Read the model definition and answer for the solid it produces. Units are mm, in the model's axes. A direction names the side the tool comes from. Coordinates: 2 decimals unless noted, no trailing zeros. Write each loop counter-clockwise with the first axis right and the second up, starting at its lowest first coordinate (ties: lowest second). Pieces come first, ordered by that corner, then holes.
(1) Section A-A on y = 2 is taken. Write down the section's boundary in (x, z), then the cut area to 3 significant figures.
(2) Find the intervals of material crossed by probe 1 along Y at (x, z) = (-3, 0.5); probe 2 along Y at (x, z) = (3.5, 2.75); probe 3 along X at (y, z) = (3.25, 0), in increasing order.
(3) Given pin 1 (1.5 mm diameter, centred on y = 5, z = -0.5, fed in from -X); pin 2 (5 mm diameter, centred on x = 4, y = 7.5, fed in from +Z); pin 3 (4 mm diameter, centred on x = 1.5, z = -1, fed in from +Y); pin 4 (0.7 mm diameter, centred on y = 3, z = 1, fed in from +X), each flat-ended and moving along its own axis, determine where each tip first touches the part or whether it passes through.
(4) Which of the six approach directions +Z, -Z, +X, -X, +Y, -Y give full straight-line access (tool end or side, diameter ignored) to faces 1 (the flat face through (0, 1, 4)), 2 (the flat face through (0, 3, -2.7)), 3 (the flat face through (-2.9, 3, 0)), 4 (the flat face through (2.9, 3, 0)), 5 (the flat face through (0, 1, -4))?
(5) The mould has two halves that part along Y. Classify faces 6 (the flat face through (-1, 0, -2)), 7 (the flat face through (2, 15, 2)), 8 (the flat face through (0, 1.8, -3)), 9 (the flat face through (5.1, 1, 0)): +Y half, -Y half, draft (parallel to the pull), parting line (faces both ways), or undercut.
from build123d import *

# Parameters (mm, degrees)
SKETCH_4_W          = 10.2
SKETCH_4_H          = 8
EXTRUDE_1_DEPTH     = 1.8
SKETCH_5_W          = 5.8
SKETCH_5_H          = 5.4
EXTRUDE_2_DEPTH     = 2.2
SKETCH_7_RX         = 3.7
SKETCH_7_RY         = 3.6
SKETCH_6_RX         = 4.4
SKETCH_6_RY         = 4.2
SKETCH_8_R          = 2
CUT_EXTRUDE_1_DEPTH = 17.442931639


with BuildPart() as part:
    # 草图4 → 凸台-拉伸1 (new body)
    with BuildSketch(Plane(origin=(0, 0, 0), x_dir=(1, 0, 0), z_dir=(0, 1, 0))):
        Rectangle(SKETCH_4_W, SKETCH_4_H)
    extrude(amount=EXTRUDE_1_DEPTH)

    # 草图5 → 凸台-拉伸2 (add)
    with BuildSketch(Plane(origin=(0, 1.8, 0), x_dir=(1, 0, 0), z_dir=(0, 1, 0))):
        Rectangle(SKETCH_5_W, SKETCH_5_H)
    extrude(amount=EXTRUDE_2_DEPTH)

    # 草图7 → 放样1 section 0
    with BuildSketch(Plane(origin=(0, 15, 0), x_dir=(-1, 0, 0), z_dir=(0, -1, 0))):
        with Locations(Location((0, 0), (0, 0, -90))):
            Ellipse(SKETCH_7_RX, SKETCH_7_RY)
    # 草图6 → 放样1 section 1
    with BuildSketch(Plane(origin=(0, 4, 0), x_dir=(1, 0, 0), z_dir=(0, 1, 0))):
        with Locations(Location((0, 0), (0, 0, 90))):
            Ellipse(SKETCH_6_RX, SKETCH_6_RY)
    loft()

    # 草图8 → 切除-拉伸1 (cut, through all)
    with BuildSketch(Plane(origin=(0, 15, 0), x_dir=(1, 0, 0), z_dir=(0, 1, 0))):
        with Locations(Location((0, 0, 0), (0, 0, 270))):
            Circle(SKETCH_8_R)
    extrude(amount=-CUT_EXTRUDE_1_DEPTH, mode=Mode.SUBTRACT)


solid = part.part
Response:
1. outline: (-2.9, -2.7) - (2.9, -2.7) - (2.9, 2.7) - (-2.9, 2.7) - close; hole circle Ø4 at (0, 0)
1. area: 18.8 mm2
2. probe 1: y = 0 to 1.8, 4 to 15
2. probe 2: y = 0 to 1.8
2. probe 3: x = -2.9 to -2, 2 to 2.9
3. pin 1: stops at x = -4.18
3. pin 2: stops at z = 3.89
3. pin 3: stops at y = 15
3. pin 4: stops at x = 2.9
4. face 1: +Z, +X, -X, -Y
4. face 2: -Z, +X, -X
4. face 3: +Z, -Z, -X
4. face 4: +Z, -Z, +X
4. face 5: -Z, +X, -X, -Y
5. face 6: -Y half
5. face 7: +Y half
5. face 8: undercut
5. face 9: draft
